Check sheet for the drawn part. Datum: minimum x, y, z corner. Units: mm. A direction names the side the tool comes from. Give positions to 0.01 mm unless a question says otherwise; leave off trailing zeros. Write each loop counter-clockwise with the first axis right and the second up, starting at its lowest first coordinate (ties: lowest second). Pieces come first, ordered by that corner, then holes.
(1) Cross-section at C-C (x = 7). Record the boundary of the cut face in (y, z).
(2) Thickness scan on line 1 along Z through (x, y) = (66, 2.5); line 2 along Y through (x, z) = (61, 31); line 3 along Z through (x, y) = (5, 29.5). Record the ranges inside material, lowest first.
(3) Tool access check on the marked faces 4, 5, 6, 7 and 8. Record the directions out of +Z, -Z, +X, -X, +Y, -Y that give a thin tool (end or side, any length) a straight path to the whole face; none if there is none.
(4) Mould release check, pull along Y, two halves, no side actions. Record for the marked faces 1, 2 and 3: +Y half, -Y half, draft (parallel to the pull), parting line (faces both ways), or undercut.
(5) Cross-section at B-B (z = 6.5). Record the boundary of the cut face in (x, y).
(6) Depth check by flat-ended pin: P1, Ø9, axis at x = 66, z = 42, coming from the -Y side; P2, Ø5, axis at x = 24, y = 6.5, coming from the +Z side; P3, Ø6, axis at x = 56.5, y = 11, coming from the +Z side; P4, Ø3, axis at x = 38, y = 6.5, coming from the -Z side. Enter the tip coordinate at first touch or a pass-through.
(7) Cross-section at A-A (x = 66). Record the boundary of the cut face in (y, z).
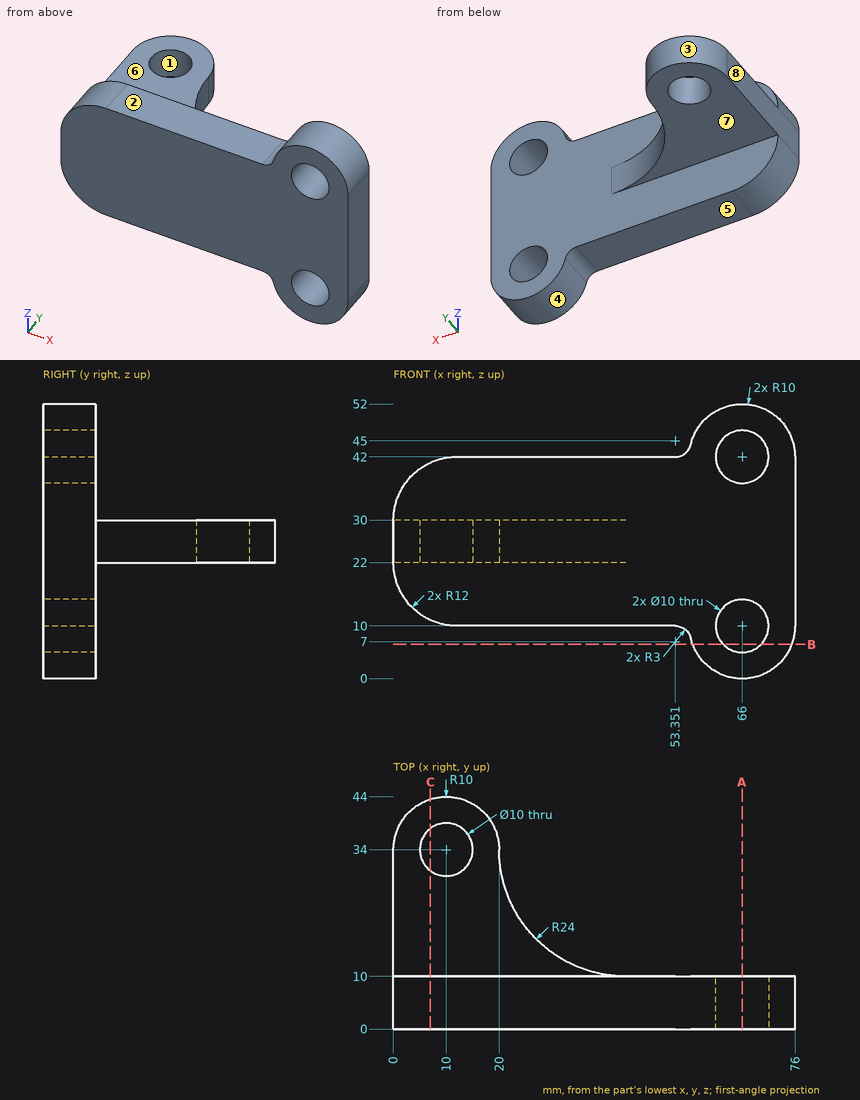
Reply:
1. outline: (0, 11.09) - (10, 11.09) - (10, 22) - (30, 22) - (30, 30) - (10, 30) - (10, 40.91) - (0, 40.91) - close; (38, 22) - (43.54, 22) - (43.54, 30) - (38, 30) - close
2. line 1: z = 0 to 5, 15 to 37, 47 to 52
2. line 2: y = 0 to 10
2. line 3: z = 22 to 30
3. face 4: -Z, +Y, -Y
3. face 5: -Z, -X, +Y, -Y
3. face 6: +Z, +X, -X, +Y
3. face 7: -Z, +X, -X, +Y
3. face 8: +Z, -Z, -X, +Y, -Y
4. face 1: undercut
4. face 2: draft
4. face 3: +Y half
5. outline: (56.63, 0) - (62.43, 0) - (62.43, 10) - (56.63, 10) - close; (69.57, 0) - (75.37, 0) - (75.37, 10) - (69.57, 10) - close
6. P1: passes through
6. P2: stops at z = 42
6. P3: stops at z = 49.45
6. P4: stops at z = 10
7. outline: (0, 0) - (10, 0) - (10, 5) - (0, 5) - close; (0, 15) - (10, 15) - (10, 37) - (0, 37) - close; (0, 47) - (10, 47) - (10, 52) - (0, 52) - close
